```python
from build123d import *

# Parameters (mm, degrees)
SKETCH_1_W      = 86
SKETCH_1_H      = 46
EXTRUDE_1_DEPTH = 2
SKETCH_2_R      = 1.5
EXTRUDE_2_DEPTH = 5.8


with BuildPart() as part:
    # 草图1 → 凸台-拉伸1 (new body)
    with BuildSketch(Plane(origin=(0, 0, 0), x_dir=(1, 0, 0), z_dir=(0, 1, 0))):
        Rectangle(SKETCH_1_W, SKETCH_1_H)
    extrude(amount=EXTRUDE_1_DEPTH)

    # 草图2 → 凸台-拉伸2 (add)
    with BuildSketch(Plane.XZ):
        with Locations(Location((-39, 19, 0), (0, 0, 270))):
            Circle(SKETCH_2_R)
        with Locations(Location((-39, -19, 0), (0, 0, 270))):
            Circle(SKETCH_2_R)
        with Locations(Location((39, 19, 0), (0, 0, 270))):
            Circle(SKETCH_2_R)
        with Locations(Location((39, -19, 0), (0, 0, 270))):
            Circle(SKETCH_2_R)
    extrude(amount=-EXTRUDE_2_DEPTH)


solid = part.part
```
The listing builds one solid part. Answer for the finished solid, in the listing's coordinates (mm). A direction names the side the tool comes from. Coordinates: 2 decimals unless noted, no trailing zeros. Write each loop counter-clockwise with the first axis right and the second up, starting at its lowest first coordinate (ties: lowest second). Pieces come first, ordered by that corner, then holes. Notation, with made-up numbers: (-10, -1.5) - (7, -1.5) arc R24 cw to (7, 12.5) - close; hole circle Ø3 at (20.25, -18). An arc over 180 degrees is marked (long way). Return JSON: item names as keys, results as strings. Group by question number.
1. A cutting plane is placed at D-D, the plane z = 4. Determine the outline of the cut face in (x, y).
2. A cutting plane is placed at C-C, the plane y = 3.45. Determine the outline of the cut face in (x, z).
3. A cutting plane is placed at A-A, the plane x = -39. Determine the outline of the cut face in (y, z).
4. Determine the mould class of faces 1 (the flat face through (-1, 1, -23)), 2 (the flat face through (39, 5.8, 19)), 3 (the cylindrical face through (38.1, 3.9, 20.2)) for opening direction Z: released by +Z, released by -Z, zero draft, split by the parting line, or undercut.
5. Which of the six approach directions +Z, -Z, +X, -X, +Y, -Y give full straight-line access (tool end or side, diameter ignored) to faces 4 (the cylindrical face through (-39.9, 3.9, -17.8)), 5 (the flat face through (39, 5.8, -19))?
6. A cutting plane is placed at B-B, the plane z = 19. Determine the outline of the cut face in (x, y), plus the area to 3 significant figures.
7. Given pin 1 (8 mm diameter, centred on x = -12, z = 11, fed in from +Y), flat-ended and moving along its own axis, determine where the tip first touches the part or whether it passes through.
8. Straight lines are drawn through the part: L1, parallel to X at y = 5.1, z = -19; L2, parallel to Y at x = -15, z = -13.5; L3, parallel to X at y = 4.85, z = 20. For each, find the intervals that lie inside material, in ascending order.
Ans:
{
 "1": {"outline": "(-43, 0) - (43, 0) - (43, 2) - (-43, 2) - close"},
 "2": {"outline": "circle Ø3 at (-39, -19); circle Ø3 at (-39, 19); circle Ø3 at (39, -19); circle Ø3 at (39, 19)"},
 "3": {"outline": "(0, -23) - (2, -23) - (2, -20.5) - (5.8, -20.5) - (5.8, -17.5) - (2, -17.5) - (2, 17.5) - (5.8, 17.5) - (5.8, 20.5) - (2, 20.5) - (2, 23) - (0, 23) - close"},
 "4": {"face 1": "released by -Z", "face 2": "zero draft", "face 3": "undercut"},
 "5": {"face 4": "+Y", "face 5": "+Z, -Z, +X, -X, +Y"},
 "6": {"outline": "(-43, 0) - (43, 0) - (43, 2) - (40.5, 2) - (40.5, 5.8) - (37.5, 5.8) - (37.5, 2) - (-37.5, 2) - (-37.5, 5.8) - (-40.5, 5.8) - (-40.5, 2) - (-43, 2) - close", "area": "195 mm²"},
 "7": {"pin 1": "y = 2"},
 "8": {"L1": "-40.5 to -37.5, 37.5 to 40.5", "L2": "0 to 2", "L3": "-40.12 to -37.88, 37.88 to 40.12"}
}
